Work out the finished part from the listing and answer in its coordinate system (mm). Face numbers are marked on the shaded views. A direction names the side the tool comes from. Round coordinates to 2 decimals unless told otherwise and drop trailing zeros. Loops run counter-clockwise (first coordinate to the right, second up) from the corner with the lowest first, then second, coordinate; pieces in that order, holes last. Notation, with made-up numbers: (76, -24.5) -> (104, -24.5) arc R17 cw to (104, 3.5) -> close; hole circle Ø10 at (64, -40). An arc over 180 degrees is marked (long way). Use one line per item in the form item = value.
```python
from build123d import *

# Parameters (mm, degrees)
F2_R     = 2.413
F4_DEPTH = 50.8
F3_R     = 2.413
F5_DEPTH = 50.8


with BuildPart() as f1:
    # F0 (on Front) → F1 (revolve)
    with BuildSketch(Plane.XZ):
        Polygon((31.75, 13.97), (31.75, 0), (33.02, 0), (33.02, 14.04055), (21.2725, 119.45055), (21.2725, 133.35), (20.0025, 133.35), (20.0025, 119.38), align=None)
    revolve(axis=Axis((0, 0, 24.955008), (0, 0, 1)))

    # F2 (on Front) → F4 (cut, symmetric)
    with BuildSketch(Plane.XZ):
        with Locations((0, 7.69055)):
            Circle(F2_R)
    extrude(amount=F4_DEPTH, both=True, mode=Mode.SUBTRACT)

    # F3 (on Right) → F5 (cut, symmetric)
    with BuildSketch(Plane.YZ):
        with Locations((0, 7.69055)):
            Circle(F3_R)
    extrude(amount=F5_DEPTH, both=True, mode=Mode.SUBTRACT)


solid = f1.part
```
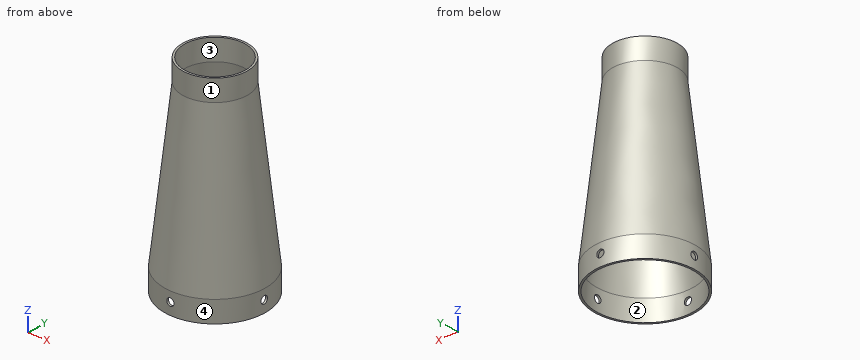
(1) For the marked faces 1 and 2, determine the directions among +Z, -Z, +X, -X, +Y, -Y from which every point of the face is accessible in a straight line to the end or side of a thin tool.
Completed:
face_1 = +Z
face_2 = -Z
(2) Find section A-A, the plane y = 0. Write down the section's boundary in (x, z).
Completed:
outline = (-33.02, 0) -> (-31.75, 0) -> (-31.75, 5.28) -> (-33.02, 5.28) -> close; (-33.02, 10.1) -> (-31.75, 10.1) -> (-31.75, 13.97) -> (-20, 119.38) -> (-20, 133.35) -> (-21.27, 133.35) -> (-21.27, 119.45) -> (-33.02, 14.04) -> close; (20, 119.38) -> (31.75, 13.97) -> (31.75, 10.1) -> (33.02, 10.1) -> (33.02, 14.04) -> (21.27, 119.45) -> (21.27, 133.35) -> (20, 133.35) -> close; (31.75, 0) -> (33.02, 0) -> (33.02, 5.28) -> (31.75, 5.28) -> close
(3) Find section C-C, the plane z = 52. Write down the section's boundary in (x, y), then the cut area to 3 significant figures.
Completed:
outline = circle Ø57.58 at (0, 0); hole circle Ø55.02 at (0, 0)
area = 226 mm2
(4) Find section D-D, the plane z = 71.5. Write down the section's boundary in (x, y), then the cut area to 3 significant figures.
Completed:
outline = circle Ø53.23 at (0, 0); hole circle Ø50.68 at (0, 0)
area = 209 mm2
(5) Consider L1, parallel to X at y = 3.5, z = 120; L2, parallel to X at y = -9.5, z = 45; L3, parallel to Y at x = 8, z = 12.5. Determine where each line is inside the solid, lowest interval first.
Completed:
L1 = -20.98 to -19.69, 19.69 to 20.98
L2 = -28 to -26.65, 26.65 to 28
L3 = -32.04 to -30.73, 30.73 to 32.04
(6) Given P1, Ø10, axis at x = -22.5, z = 71, coming from the +Y side; P2, Ø3, axis at y = 0, z = 7.69, coming from the -X side; P3, Ø1, axis at x = 17.5, z = 34, coming from the +Y side; P4, Ø6, axis at x = 16.5, y = 26, coming from the -Z side, each flat-ended and moving along its own axis, determine where each tip first touches the part or whether it passes through.
Completed:
P1 = 20.19
P2 = through
P3 = 25.68
P4 = 0
(7) For a pull along X with two mould halves and no side action, classify the marked faces 3 and 4 as +X half, -X half, draft (parallel to the pull), parting line (faces both ways), or undercut.
Completed:
face_3 = undercut
face_4 = parting line
